Design review of the part shown in the three views and the two pictorial views. Dimensions are in mm from the part's minimum x, y and z. Give positions to 0.01 mm unless a question says otherwise; leave off trailing zeros. Loops run counter-clockwise (first coordinate to the right, second up) from the corner with the lowest first, then second, coordinate; pieces in that order, holes last. Notation, with made-up numbers: (67.5, -17) -> (115.5, -17) arc R12 ccw to (115.5, -13) -> close; hole circle Ø11 at (36, 66.5). An arc over 180 degrees is marked (long way). Use CSV: the item, a comma, the result in double quotes. Start each with the question number.
Item 1: Wall thickness on line 1 along Y through (x, z) = (12, 7); line 2 along Y through (x, z) = (68, 4.75); line 3 along X through (y, z) = (39.5, 5): over which ranges is each line inside the solid? List them lowest first. Write a range as from..to.
Item 2: We need section A-A (x = 12). State the section outline as (y, z) points, plus the area to 3 significant figures.
Item 3: We need section C-C (x = 68). State the section outline as (y, z) points, plus the area to 3 significant figures.
Item 4: We need section D-D (y = 45). State the section outline as (x, z) points.
Item 5: We need section B-B (z = 5). State the section outline as (x, y) points (1 decimal), plus the area to 3 significant figures.
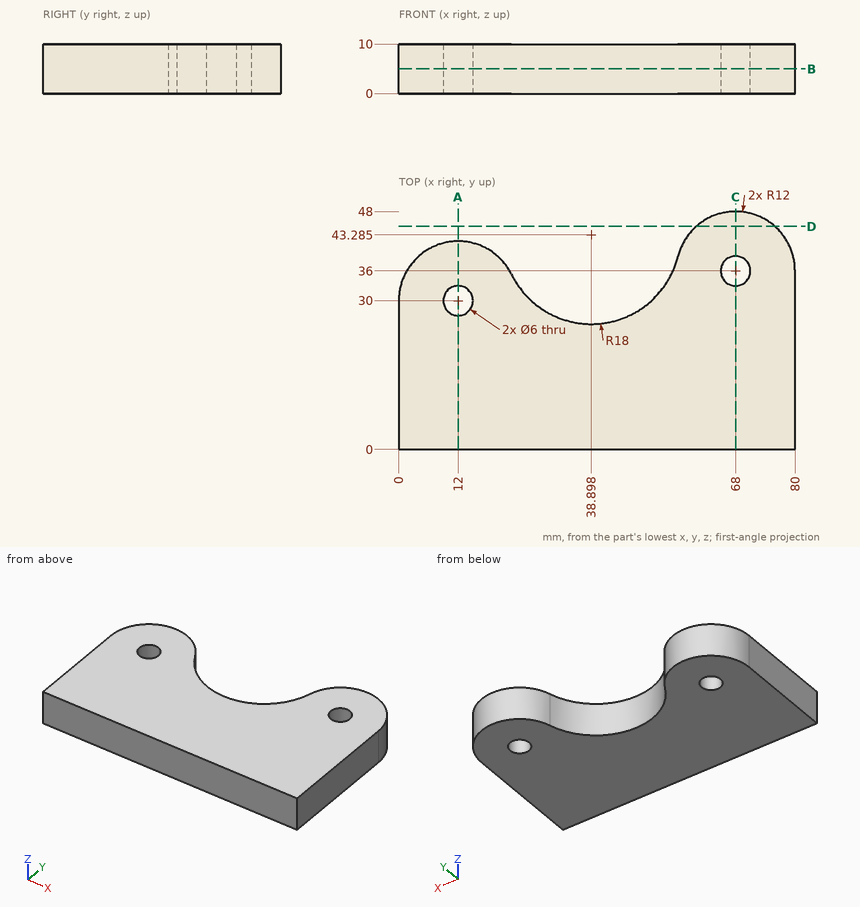
Results found:
1,line 1,"0..27, 33..42"
1,line 2,"0..33, 39..48"
1,line 3,"4.67..19.33, 56.52..79.48"
2,outline,"(0, 0) -> (27, 0) -> (27, 10) -> (0, 10) -> close; (33, 0) -> (42, 0) -> (42, 10) -> (33, 10) -> close"
2,area,"360 mm²"
3,outline,"(0, 0) -> (33, 0) -> (33, 10) -> (0, 10) -> close; (39, 0) -> (48, 0) -> (48, 10) -> (39, 10) -> close"
3,area,"420 mm²"
4,outline,"(60.06, 0) -> (75.94, 0) -> (75.94, 10) -> (60.06, 10) -> close"
5,outline,"(0, 0) -> (80, 0) -> (80, 36) arc R12 ccw to (56.4, 38.9) arc R18 cw to (22.8, 35.3) arc R12 ccw to (0, 30) -> close; hole circle Ø6 at (12, 30); hole circle Ø6 at (68, 36)"
5,area,"2,880 mm²"
